```python
from build123d import *

# Parameters (mm, degrees)
SKETCH1_W           = 289.69
SKETCH1_H           = 12.7
SKETCH1_R           = 2.49
BOSS_EXTRUDE1_DEPTH = 6.35
FILLET1_R           = 2.54
SKETCH3_W           = 289.687
SKETCH3_H           = 38.1
SKETCH3_R           = 2.4892
BOSS_EXTRUDE2_DEPTH = 6.35


with BuildPart() as part:
    # Sketch1 → Boss-Extrude1 (new body)
    # profile 1 of 3: a face of its own
    with BuildSketch(Plane(origin=(0, 0, 0), x_dir=(1, 0, 0), z_dir=(0, 1, 0))):
        with Locations((0, -25.4)):
            Rectangle(SKETCH1_W, SKETCH1_H)
        with Locations(Location((138.495, -25.4, 0), (0, 0, 270))):
            Circle(SKETCH1_R, mode=Mode.SUBTRACT)
        with Locations(Location((0, -25.4, 0), (0, 0, 270))):
            Circle(SKETCH1_R, mode=Mode.SUBTRACT)
    # profile 2 of 3: a face of its own
    with BuildSketch(Plane(origin=(0, 0, 0), x_dir=(1, 0, 0), z_dir=(0, 1, 0))):
        Polygon((-144.845, 31.75), (-157.545, 31.75), (-157.545, -31.75), (-144.845, -31.75), (-144.845, -19.05), (-144.845, 19.05), align=None)
        with Locations(Location((-151.195, -25.4, 0), (0, 0, 270))):
            Circle(SKETCH1_R, mode=Mode.SUBTRACT)
        with Locations(Location((-151.195, 25.4, 0), (0, 0, 270))):
            Circle(SKETCH1_R, mode=Mode.SUBTRACT)
    # profile 3 of 3: a face of its own
    with BuildSketch(Plane(origin=(0, 0, 0), x_dir=(1, 0, 0), z_dir=(0, 1, 0))):
        with Locations((0, 25.4)):
            Rectangle(SKETCH1_W, SKETCH1_H)
        with Locations(Location((138.495, 25.4, 0), (0, 0, 270))):
            Circle(SKETCH1_R, mode=Mode.SUBTRACT)
        with Locations(Location((0, 25.4, 0), (0, 0, 270))):
            Circle(SKETCH1_R, mode=Mode.SUBTRACT)
    extrude(amount=BOSS_EXTRUDE1_DEPTH)

    # Fillet1
    fillet1_edges = [part.edges().sort_by_distance(p)[0] for p in [
        (144.845, 3.175, 31.75),
        (-157.545, 3.175, 31.75),
        (-157.545, 3.175, -31.75),
        (144.845, 3.175, -31.75),
    ]]
    fillet(fillet1_edges, radius=FILLET1_R)

    # Sketch3 → Boss-Extrude2 (add)
    with BuildSketch(Plane(origin=(0, 6.35, 0), x_dir=(1, 0, 0), z_dir=(0, 1, 0))):
        with Locations((-0.0015, 0)):
            Rectangle(SKETCH3_W, SKETCH3_H)
        with Locations(Location((-137.7076, 13.4874, 0), (0, 0, 270))):
            Circle(SKETCH3_R, mode=Mode.SUBTRACT)
        with Locations(Location((-137.733, -13.4874, 0), (0, 0, 270))):
            Circle(SKETCH3_R, mode=Mode.SUBTRACT)
        with Locations(Location((-47.6392, -13.4874, 0), (0, 0, 270))):
            Circle(SKETCH3_R, mode=Mode.SUBTRACT)
        with Locations(Location((-47.6392, 13.4874, 0), (0, 0, 270))):
            Circle(SKETCH3_R, mode=Mode.SUBTRACT)
        with Locations(Location((47.6108, 13.4874, 0), (0, 0, 270))):
            Circle(SKETCH3_R, mode=Mode.SUBTRACT)
        with Locations(Location((47.6108, -13.4874, 0), (0, 0, 270))):
            Circle(SKETCH3_R, mode=Mode.SUBTRACT)
        with Locations(Location((137.6792, 13.4874, 0), (0, 0, 270))):
            Circle(SKETCH3_R, mode=Mode.SUBTRACT)
        with Locations(Location((137.6792, -13.4874, 0), (0, 0, 270))):
            Circle(SKETCH3_R, mode=Mode.SUBTRACT)
    extrude(amount=-BOSS_EXTRUDE2_DEPTH)


solid = part.part
```
Could you check a few things on this model? Use its own coordinates, in mm. Round coordinates to 2 decimals unless told otherwise and drop trailing zeros. Loops run counter-clockwise (first coordinate to the right, second up) from the corner with the lowest first, then second, coordinate; pieces in that order, holes last. Notation, with made-up numbers: M 82.5,-33 L 90.5,-33 A17 ccw 90.5,-4 Z; hole C 70,-3 d10. An arc over 180 degrees is marked long. Answer as CSV lines item,"result".
1) If I drill on probe 1 along X at (y, z) = (3.5, 25.4) (3 decimals); probe 2 along X at (y, z) = (2.5, -26.5) (3 decimals); probe 3 along X at (y, z) = (2.5, 15) (3 decimals), over which ranges is the centre line in solid material (lowest first)?
From the geometry:
probe 1,"-157.545 to -153.685, -148.705 to -2.49, 2.49 to 136.005, 140.985 to 144.845"
probe 2,"-157.545 to -153.429, -148.961 to -2.234, 2.234 to 136.261, 140.729 to 144.845"
probe 3,"-157.545 to -139.71, -135.756 to -49.616, -45.662 to 45.634, 49.588 to 135.702, 139.656 to 144.842"
2) Imagine slicing it at A-A on x = 0. List the corners of the cut face in (y, z) for me.
From the geometry:
outline,"M 0,-31.75 L 6.35,-31.75 L 6.35,-27.89 L 0,-27.89 Z; M 0,-22.91 L 6.35,-22.91 L 6.35,22.91 L 0,22.91 Z; M 0,27.89 L 6.35,27.89 L 6.35,31.75 L 0,31.75 Z"
3) Imagine slicing it at B-B on z = -25.4. List the corners of the cut face in (x, y) for me (3 decimals).
From the geometry:
outline,"M -157.545,0 L -153.685,0 L -153.685,6.35 L -157.545,6.35 Z; M -148.705,0 L -2.49,0 L -2.49,6.35 L -148.705,6.35 Z; M 2.49,0 L 136.005,0 L 136.005,6.35 L 2.49,6.35 Z; M 140.985,0 L 144.845,0 L 144.845,6.35 L 140.985,6.35 Z"
4) We'd pull the mould along Z, two halves only. Please class faces 1 (the flat face through (144.845, 3, 24)), 2 (the cylindrical face through (139.36, 3.22, 11.65)), 3 (the flat face through (-8, 3, 31.75)): released by +Z, released by -Z, zero draft, split by the parting line, or undercut.
From the geometry:
face 1,"zero draft"
face 2,"undercut"
face 3,"released by +Z"
